from build123d import *

# Parameters (mm, degrees)
ESQUISSE1_W                  = 70
ESQUISSE1_H                  = 70
BOSS_EXTRU_1_DEPTH           = 64
ESQUISSE2_W                  = 30.4
ESQUISSE2_H                  = 19.8
ESQUISSE2_H_2                = 30.4
ESQUISSE2_W_2                = 19.8
ENL_V_MAT_EXTRU_1_DEPTH      = 50
ESQUISSE5_W                  = 3
ESQUISSE5_H                  = 2
ENL_V_MAT_EXTRU_3_DEPTH      = 71
ESQUISSE6_W                  = 2
ESQUISSE6_H                  = 3
ENL_V_MAT_EXTRU_4_DEPTH      = 71
ESQUISSE7_R                  = 1
ENL_V_MAT_EXTRU_5_DEPTH      = 65
ENL_V_MAT_EXTRU_7_DEPTH      = 10
BOSS_EXTRU_2_DEPTH           = 3.8
ESQUISSE10_W                 = 27
ESQUISSE10_H                 = 18.1
ENL_V_MAT_EXTRU_8_DEPTH      = 10
ESQUISSE11_R                 = 1.25
ENL_V_MAT_EXTRU_9_DEPTH      = 15
R_P_TITION_CIRCULAIRE1_COUNT = 4


with BuildPart() as part:
    # Esquisse1 → Boss.-Extru.1 (new body)
    with BuildSketch(Plane.XY):
        with Locations((-35, 35)):
            Rectangle(ESQUISSE1_W, ESQUISSE1_H)
    extrude(amount=BOSS_EXTRU_1_DEPTH)

    # Esquisse2 → Enlèv. mat.-Extru.1 (cut)
    with BuildSketch(Plane.XY.offset(64)):
        with Locations((-35, 60.1)):
            Rectangle(ESQUISSE2_W, ESQUISSE2_H)
        with Locations((-35, 35)):
            Rectangle(ESQUISSE2_W, ESQUISSE2_H_2)
        with Locations((-9.9, 35)):
            Rectangle(ESQUISSE2_W_2, ESQUISSE2_H_2)
        with Locations((-60.1, 35)):
            Rectangle(ESQUISSE2_W_2, ESQUISSE2_H_2)
        with Locations((-35, 9.9)):
            Rectangle(ESQUISSE2_W, ESQUISSE2_H)
    extrude(amount=-ENL_V_MAT_EXTRU_1_DEPTH, mode=Mode.SUBTRACT)

    # Esquisse5 → Enlèv. mat.-Extru.3 (cut, through all)
    with BuildSketch(Plane.ZY.offset(70)):
        with Locations((59.5, 69)):
            Rectangle(ESQUISSE5_W, ESQUISSE5_H)
        with Locations((59.5, 1)):
            Rectangle(ESQUISSE5_W, ESQUISSE5_H)
    extrude(amount=-ENL_V_MAT_EXTRU_3_DEPTH, mode=Mode.SUBTRACT)

    # Esquisse6 → Enlèv. mat.-Extru.4 (cut, through all)
    with BuildSketch(Plane(origin=(0, 70, 0), x_dir=(1, 0, 0), z_dir=(0, 1, 0))):
        with Locations((-69, -59.5)):
            Rectangle(ESQUISSE6_W, ESQUISSE6_H)
    extrude(amount=-ENL_V_MAT_EXTRU_4_DEPTH, mode=Mode.SUBTRACT)

    # Esquisse7 → Enlèv. mat.-Extru.5 (cut, through all)
    with BuildSketch(Plane.XY.offset(64)):
        with Locations((-52.2, 17.8)):
            Circle(ESQUISSE7_R)
    enl_v_mat_extru_5 = extrude(amount=-ENL_V_MAT_EXTRU_5_DEPTH, mode=Mode.SUBTRACT)

    # Esquisse8 → Enlèv. mat.-Extru.7 (cut)
    with BuildSketch(Plane(origin=(0, 0, 0), x_dir=(-1, 0, 0), z_dir=(0, 0, -1))):
        with BuildLine():
            Line((60.2, 0), (60.2, 17.8))
            ThreePointArc((60.2, 17.8), (52.2, 9.8), (44.2, 17.8))
            Line((44.2, 17.8), (44.2, 0))
            Line((44.2, 0), (60.2, 0))
        make_face()
        with BuildLine():
            ThreePointArc((44.2, 17.8), (52.2, 9.8), (60.2, 17.8))
            Line((60.2, 17.8), (53.2, 17.8))
            ThreePointArc((53.2, 17.8), (52.2, 16.8), (51.2, 17.8))
            Line((51.2, 17.8), (44.2, 17.8))
        make_face()
        with BuildLine():
            Line((53.2, 17.8), (60.2, 17.8))
            ThreePointArc((60.2, 17.8), (52.2, 25.8), (44.2, 17.8))
            Line((44.2, 17.8), (51.2, 17.8))
            ThreePointArc((51.2, 17.8), (52.2, 18.8), (53.2, 17.8))
        make_face()
    enl_v_mat_extru_7 = extrude(amount=-ENL_V_MAT_EXTRU_7_DEPTH, mode=Mode.SUBTRACT)

    # Esquisse9 → Boss.-Extru.2 (add)
    with BuildSketch(Plane(origin=(0, 0, 0), x_dir=(-1, 0, 0), z_dir=(0, 0, -1))):
        with BuildLine():
            Line((46.2, 0), (46.2, 17.8))
            ThreePointArc((46.2, 17.8), (52.2, 23.8), (58.2, 17.8))
            Line((58.2, 17.8), (58.2, 0))
            Line((58.2, 0), (60.2, 0))
            Line((60.2, 0), (60.2, 17.8))
            Line((60.2, 17.8), (60.175717696, 28.742363645))
            Line((60.175717696, 28.742363645), (44.2, 28.742363645))
            Line((44.2, 28.742363645), (44.2, 0))
            Line((44.2, 0), (46.2, 0))
        make_face()
    extrude(amount=-BOSS_EXTRU_2_DEPTH)

    # Esquisse10 → Enlèv. mat.-Extru.8 (cut)
    with BuildSketch(Plane(origin=(0, 0, 0), x_dir=(-1, 0, 0), z_dir=(0, 0, -1))):
        with Locations((52.2, 9.05)):
            Rectangle(ESQUISSE10_W, ESQUISSE10_H)
    enl_v_mat_extru_8 = extrude(amount=-ENL_V_MAT_EXTRU_8_DEPTH, mode=Mode.SUBTRACT)

    # Esquisse11 → Enlèv. mat.-Extru.9 (cut)
    with BuildSketch(Plane.XZ.offset(-18.1)):
        with Locations(Location((-41.7, 7, 0), (0, 0, 270))):  # turned: the seam where the file's is
            Circle(ESQUISSE11_R)
        with Locations(Location((-62.7, 7, 0), (0, 0, 270))):  # turned: the seam where the file's is
            Circle(ESQUISSE11_R)
    extrude(amount=-ENL_V_MAT_EXTRU_9_DEPTH, mode=Mode.SUBTRACT)

    # Répétition circulaire1: Enlèv. mat.-Extru.5, Enlèv. mat.-Extru.7, Enlèv. mat.-Extru.8 ×4 about axis
    r_p_tition_circulaire1_axis = Axis((-35, 35, 0), (0, 0, 1))
    add([enl_v_mat_extru_5.rotate(r_p_tition_circulaire1_axis, i * 360 / R_P_TITION_CIRCULAIRE1_COUNT) for i in range(1, R_P_TITION_CIRCULAIRE1_COUNT)], mode=Mode.SUBTRACT)
    add([enl_v_mat_extru_7.rotate(r_p_tition_circulaire1_axis, i * 360 / R_P_TITION_CIRCULAIRE1_COUNT) for i in range(1, R_P_TITION_CIRCULAIRE1_COUNT)], mode=Mode.SUBTRACT)
    add([enl_v_mat_extru_8.rotate(r_p_tition_circulaire1_axis, i * 360 / R_P_TITION_CIRCULAIRE1_COUNT) for i in range(1, R_P_TITION_CIRCULAIRE1_COUNT)], mode=Mode.SUBTRACT)


solid = part.part
Geometry: final body of the model. Coordinates: model frame, mm. A direction names the side the tool comes from. Give positions to 0.01 mm unless a question says otherwise; leave off trailing zeros. Write each loop counter-clockwise with the first axis right and the second up, starting at its lowest first coordinate (ties: lowest second). Pieces come first, ordered by that corner, then holes. Notation, with made-up numbers: M -28,32.25 L 12,32.25 A24 ccw 12,71.25 Z; hole C -38.5,28 d2. An arc over 180 degrees is marked long. Answer in a Markdown table with one row per item. Add a question column.
(1) Section C-C on x = -27.5. Return loops of the section in (y, z).
(2) Mould query, pull axis X, two halves, no side actions, for faces 4 (the flat face through (-68.2, 64.5, 61)), 5 (the cylindrical face through (-25.8, 17.63, 4.93)), 6 (the cylindrical face through (-53.2, 17.8, 37.4)). Classes: +X half, -X half, draft (parallel to the pull), parting line (faces both ways), or undercut.
(3) Section D-D on x = -54.5. Return loops of the section in (y, z).
(4) First-contact query: pin 1 (2.5 mm diameter, centred on x = -17.8, y = 52.2, fed in from -Z); pin 2 (4 mm diameter, centred on x = -62.7, z = 7, fed in from -Y); pin 3 (4 mm diameter, centred on x = -53, y = 34.5, fed in from +Z). Flat tips, straight axial feed; report the tip coordinate or a pass-through.
(5) Ray query, line 1 (X direction, y = 52, z = 40); line 2 (Y direction, x = -17.8, z = 40); line 3 (Y direction, x = -17, z = 30). Return the intervals inside material, ascending.
(6) Reachability of faces 1 (the flat face through (-19.8, 60, 39)), 2 (the flat face through (-9, 4.3, 5)), 3 (the flat face through (-61, 65.7, 5)) from +Z, -Z, +X, -X, +Y, -Y: full face, straight path, thin tool, end or side. Return the list, or none.
(7) Section A-A on z = 37. Return loops of the section in (x, y).
(8) Section B-B on y = 58. Return loops of the section in (x, z).
Result set:
| question | item | result |
|---|---|---|
| 1 | outline | M 0,0 L 51.9,0 L 51.9,10 L 70,10 L 70,14 L 0,14 Z |
| 2 | face 4 | draft |
| 2 | face 5 | +X half |
| 2 | face 6 | undercut |
| 3 | outline | M 0,10 L 25.46,10 L 25.46,3.8 L 23.34,3.8 L 23.34,0 L 38.7,0 L 38.7,10 L 65.7,10 L 65.7,0 L 70,0 L 70,58 L 68,58 L 68,61 L 70,61 L 70,64 L 50.2,64 L 50.2,14 L 19.8,14 L 19.8,64 L 0,64 L 0,61 L 2,61 L 2,58 L 0,58 Z |
| 4 | pin 1 | stops at z = 10 |
| 4 | pin 2 | stops at y = 18.1 |
| 4 | pin 3 | stops at z = 14 |
| 5 | line 1 | x = -70 to -53.18, -51.22 to -50.2, -19.8 to -18.78, -16.82 to 0 |
| 5 | line 2 | y = 0 to 16.8, 18.8 to 19.8, 50.2 to 51.2, 53.2 to 70 |
| 5 | line 3 | y = 0 to 17.2, 18.4 to 19.8, 50.2 to 51.6, 52.8 to 70 |
| 6 | face 1 | +Z, +Y, -Y |
| 6 | face 2 | -Z, +X |
| 6 | face 3 | -Z, -X |
| 7 | outline | M -70,0 L -50.2,0 L -50.2,19.8 L -70,19.8 Z; M -70,50.2 L -50.2,50.2 L -50.2,70 L -70,70 Z; M -19.8,0 L 0,0 L 0,19.8 L -19.8,19.8 Z; M -19.8,50.2 L 0,50.2 L 0,70 L -19.8,70 Z; hole C -52.2,17.8 d2; hole C -52.2,52.2 d2; hole C -17.8,17.8 d2; hole C -17.8,52.2 d2 |
| 8 | outline | M -70,10 L -46.69,10 L -46.69,0 L -31.3,0 L -31.3,10 L -4.3,10 L -4.3,0 L 0,0 L 0,64 L -19.8,64 L -19.8,14 L -50.2,14 L -50.2,64 L -70,64 L -70,61 L -68,61 L -68,58 L -70,58 Z |
